Solid Edge part; units mm, degrees
sketch "Sketch1" plane through (0, 0, 0) normal (0, 0, 1) x (1, 0, 0)
  circle A0 centre (0, 0) radius 10.5
extrude "Ajout_matière_1" add sketch "Sketch1" along normal blind 11.5
sketch "Sketch2" plane through (0, 0, 11.5) normal (0, 0, 1) x (1, 0, 0)
  circle A0 centre (0, 10.5) radius 0.998
extrude "Cutout1" cut sketch "Sketch2" against normal through all
pattern_circular "Pattern1" count 25 over 360 about axis through (0, 0, 11.5) along (0, 0, -1) of "Cutout1"
sketch "Sketch3" plane through (0, -0.0199, 11.5) normal (0, 0, 1) x (0, -1, 0)
  circle A0 centre (-0.0199, 0) radius 1.9207
extrude "Cutout2" cut sketch "Sketch3" along normal through all and the other way through all
properties material "Nylon, usage général"
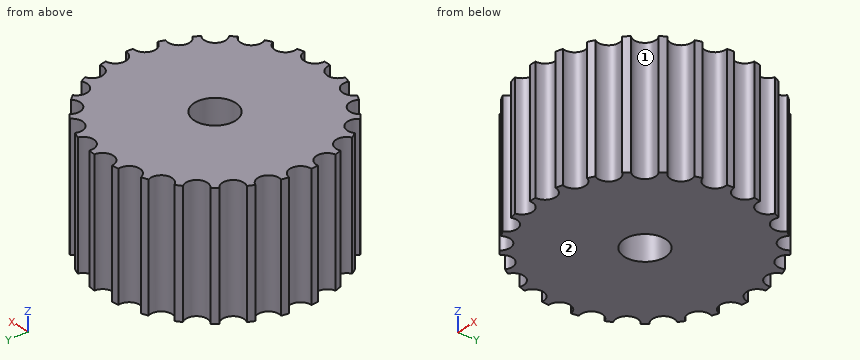
Work out the finished part from the listing and answer in its coordinate system (mm). Face numbers are marked on the shaded views. Round coordinates to 2 decimals unless told otherwise and drop trailing zeros. Write each loop counter-clockwise with the first axis right and the second up, starting at its lowest first coordinate (ties: lowest second). Pieces come first, ordered by that corner, then holes. Notation, with made-up numbers: (49.25, -15) -> (78.25, -15) arc R21 cw to (78.25, 12) -> close; hole circle Ø1 at (-26.75, 8). An arc over 180 degrees is marked (long way). Write each question's results on one line, items separated by ' | '.
1) Consider line 1 along X through (y, z) = (4.5, 9.5); line 2 along X through (y, z) = (0, 6.25); line 3 along Y through (x, z) = (0.5, 2.75). Determine where each line is inside the solid, lowest interval first. Write a range as [from, to].
Findings:
line 1: x = [-9.49, 9.49] | line 2: x = [-9.73, -1.92], [1.92, 9.73] | line 3: y = [-9.84, -1.85], [1.85, 9.64]
2) Flat-ended cylindrical pins translate along their axes: pin 1 (1 mm diameter, centred on y = 6.5, z = 10, fed in from -X); pin 2 (2 mm diameter, centred on x = 4.5, z = 6.5, fed in from -Y); pin 3 (1 mm diameter, centred on x = -7.5, z = 5, fed in from +Y). Find the tip coordinate at first contact, or state that the pin passes through.
Findings:
pin 1: stops at x = -8.29 | pin 2: stops at y = -9.35 | pin 3: stops at y = 6.94
3) The part is cut by section C-C (y = -4). Write down the section's boundary in (x, z).
Findings:
outline: (-8.62, 0) -> (8.62, 0) -> (8.62, 11.5) -> (-8.62, 11.5) -> close
4) For a pull along X with two mould halves and no side action, classify the marked faces 1 and 2 as +X half, -X half, draft (parallel to the pull), parting line (faces both ways), or undercut.
Findings:
face 1: undercut | face 2: draft
5) The part is cut by section B-B (y = 0). Write down the section's boundary in (x, z), and give its area (3 significant figures).
Findings:
outline: (-9.73, 0) -> (-1.92, 0) -> (-1.92, 11.5) -> (-9.73, 11.5) -> close; (1.92, 0) -> (9.73, 0) -> (9.73, 11.5) -> (1.92, 11.5) -> close | area: 180 mm²
6) The part is cut by section A-A (x = 0). Write down the section's boundary in (y, z).
Findings:
outline: (-10.5, 0) -> (-1.92, 0) -> (-1.92, 11.5) -> (-10.5, 11.5) -> close; (1.92, 0) -> (9.5, 0) -> (9.5, 11.5) -> (1.92, 11.5) -> close
